```python
from build123d import *

# Parameters (mm, degrees)
SKETCH_1_W          = 47.691438342
SKETCH_1_H          = 48.077140414
EXTRUDE_2_DEPTH     = 10
SKETCH_4_W          = 47.691438342
SKETCH_4_H          = 48.077140414
EXTRUDE_3_DEPTH     = 3
CUT_EXTRUDE_1_DEPTH = 3
SKETCH_6_R          = 11.5
CUT_EXTRUDE_2_DEPTH = 3
CHAMFER_1_SIZE      = 5
SKETCH_7_W          = 26
SKETCH_7_H          = 13
EXTRUDE_4_DEPTH     = 50
SKETCH_8_W          = 20
SKETCH_8_H          = 40
CUT_EXTRUDE_3_DEPTH = 8
SKETCH_9_W          = 20
SKETCH_9_H          = 8
EXTRUDE_5_DEPTH     = 1.93
SKETCH_10_W         = 11.5
SKETCH_10_H         = 13
SKETCH_10_W_2       = 18
EXTRUDE_6_DEPTH     = 25
FILLET_1_R          = 2
SKETCH_11_R         = 2.5
CUT_EXTRUDE_4_DEPTH = 25


with BuildPart() as part:
    # 草图1 → 凸台-拉伸2 (new body)
    with BuildSketch(Plane(origin=(0, 0, 0), x_dir=(1, 0, 0), z_dir=(0, 1, 0))):
        Rectangle(SKETCH_1_W, SKETCH_1_H)
        Polygon((-21.154280829, -15.961429793), (-16.154280829, -20.961429793), (15.845719171, -20.961429793), (20.845719171, -15.961429793), (20.845719171, 16.038570207), (15.845719171, 21.038570207), (-16.154280829, 21.038570207), (-21.154280829, 16.038570207), align=None, mode=Mode.SUBTRACT)
    extrude(amount=EXTRUDE_2_DEPTH)

    # 草图4 → 凸台-拉伸3 (add)
    with BuildSketch(Plane(origin=(0, 10, 0), x_dir=(1, 0, 0), z_dir=(0, 1, 0))):
        Rectangle(SKETCH_4_W, SKETCH_4_H)
    extrude(amount=EXTRUDE_3_DEPTH)

    # 草图5 → 切除-拉伸1 (cut)
    with BuildSketch(Plane.XZ.offset(-10)):
        with BuildLine():
            ThreePointArc((-13.95, -15.5), (-14.403984489, -14.403984489), (-15.5, -13.95))
            Line((-15.5, -13.95), (-15.5, -15.5))
            Line((-15.5, -15.5), (-13.95, -15.5))
        make_face()
        with BuildLine():
            Line((-15.5, -15.5), (-15.5, -13.95))
            ThreePointArc((-15.5, -13.95), (-16.596015511, -16.596015511), (-13.95, -15.5))
            Line((-13.95, -15.5), (-15.5, -15.5))
        make_face()
        with BuildLine():
            ThreePointArc((17.05, -15.5), (16.596015511, -14.403984489), (15.5, -13.95))
            Line((15.5, -13.95), (15.5, -15.5))
            Line((15.5, -15.5), (13.95, -15.5))
            ThreePointArc((13.95, -15.5), (15.5, -17.05), (17.05, -15.5))
        make_face()
        with BuildLine():
            Line((15.5, -15.5), (15.5, -13.95))
            ThreePointArc((15.5, -13.95), (14.403984489, -14.403984489), (13.95, -15.5))
            Line((13.95, -15.5), (15.5, -15.5))
        make_face()
        with BuildLine():
            ThreePointArc((17.05, 15.5), (15.5, 17.05), (13.95, 15.5))
            Line((13.95, 15.5), (15.5, 15.5))
            Line((15.5, 15.5), (15.5, 13.95))
            ThreePointArc((15.5, 13.95), (16.596015511, 14.403984489), (17.05, 15.5))
        make_face()
        with BuildLine():
            Line((15.5, 15.5), (13.95, 15.5))
            ThreePointArc((13.95, 15.5), (14.403984489, 14.403984489), (15.5, 13.95))
            Line((15.5, 13.95), (15.5, 15.5))
        make_face()
        with BuildLine():
            ThreePointArc((-15.5, 13.95), (-14.403984489, 14.403984489), (-13.95, 15.5))
            Line((-13.95, 15.5), (-15.5, 15.5))
            Line((-15.5, 15.5), (-15.5, 13.95))
        make_face()
        with BuildLine():
            Line((-15.5, 15.5), (-13.95, 15.5))
            ThreePointArc((-13.95, 15.5), (-16.596015511, 16.596015511), (-15.5, 13.95))
            Line((-15.5, 13.95), (-15.5, 15.5))
        make_face()
    extrude(amount=-CUT_EXTRUDE_1_DEPTH, mode=Mode.SUBTRACT)

    # 草图6 → 切除-拉伸2 (cut)
    with BuildSketch(Plane(origin=(0, 13, 0), x_dir=(1, 0, 0), z_dir=(0, 1, 0))):
        with Locations(Location((0, 0, 0), (0, 0, 270))):
            Circle(SKETCH_6_R)
    extrude(amount=-CUT_EXTRUDE_2_DEPTH, mode=Mode.SUBTRACT)

    # 倒角1
    chamfer_1_edges = [part.edges().sort_by_distance(p)[0] for p in [
        (23.845719171, 6.5, -24.038570207),
        (23.845719171, 6.5, 24.038570207),
        (-23.845719171, 6.5, 24.038570207),
        (-23.845719171, 6.5, -24.038570207),
    ]]
    chamfer(chamfer_1_edges, length=CHAMFER_1_SIZE)

    # 草图7 → 凸台-拉伸4 (add)
    with BuildSketch(Plane(origin=(0, 0, -24.038570207), x_dir=(-1, 0, 0), z_dir=(0, 0, -1))):
        with Locations((0, 6.5)):
            Rectangle(SKETCH_7_W, SKETCH_7_H)
    extrude(amount=EXTRUDE_4_DEPTH)

    # 草图8 → 切除-拉伸3 (cut)
    with BuildSketch(Plane(origin=(0, 13, 0), x_dir=(1, 0, 0), z_dir=(0, 1, 0))):
        with Locations((0, 54.038570207)):
            Rectangle(SKETCH_8_W, SKETCH_8_H)
    extrude(amount=-CUT_EXTRUDE_3_DEPTH, mode=Mode.SUBTRACT)

    # 草图9 → 凸台-拉伸5 (add)
    with BuildSketch(Plane(origin=(0, 0, -34.038570207), x_dir=(-1, 0, 0), z_dir=(0, 0, -1))):
        with Locations((0, 9)):
            Rectangle(SKETCH_9_W, SKETCH_9_H)
    extrude(amount=EXTRUDE_5_DEPTH)

    # 草图10 → 凸台-拉伸6 (add)
    with BuildSketch(Plane(origin=(13, 0, 0), x_dir=(0, 0, -1), z_dir=(1, 0, 0))):
        with Locations((29.788570207, 6.5)):
            Rectangle(SKETCH_10_W, SKETCH_10_H)
        with Locations((65.038570207, 6.5)):
            Rectangle(SKETCH_10_W_2, SKETCH_10_H)
    extrude(amount=EXTRUDE_6_DEPTH)

    # 圆角1
    fillet_1_edges = [part.edges().sort_by_distance(p)[0] for p in [
        (-13, 0, -49.038570207),
        (13, 6.5, -35.538570207),
        (38, 6.5, -24.038570207),
        (38, 6.5, -35.538570207),
        (13, 6.5, -56.038570207),
        (38, 6.5, -56.038570207),
        (38, 6.5, -74.038570207),
    ]]
    fillet(fillet_1_edges, radius=FILLET_1_R)

    # 草图11 → 切除-拉伸4 (cut)
    with BuildSketch(Plane(origin=(0, 5, 0), x_dir=(1, 0, 0), z_dir=(0, 1, 0))):
        with Locations(Location((0, 64.038570207, 0), (0, 0, 270))):
            Circle(SKETCH_11_R)
        with Locations(Location((0, 49.038570207, 0), (0, 0, 270))):
            Circle(SKETCH_11_R)
    extrude(amount=-CUT_EXTRUDE_4_DEPTH, mode=Mode.SUBTRACT)


solid = part.part
```
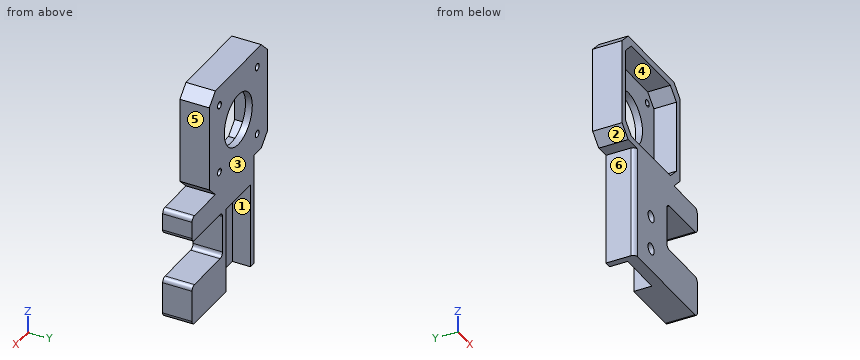
Can you work these out from the model? Positions are in its coordinate system, mm. Face numbers are marked on the shaded views. A direction names the side the tool comes from. Give positions to 0.01 mm unless a question says otherwise; leave off trailing zeros. Loops run counter-clockwise (first coordinate to the right, second up) from the corner with the lowest first, then second, coordinate; pieces in that order, holes last. Notation, with made-up numbers: M 30.25,-18 L 78.25,-18 A26 cw 78.25,21 Z; hole C 12,67.5 d11. An arc over 180 degrees is marked long. Answer in a Markdown table with one row per item.
1. Thinking about a two-plate mould opening in X: for the marked faces 1, 2 and 3, which applies, released by +X, released by -X, zero draft, split by the parting line, or undercut?
Taken from the geometry:
| item | result |
|---|---|
| face 1 | undercut |
| face 2 | released by -X |
| face 3 | zero draft |
2. Which directions (+Z, -Z, +X, -X, +Y, -Y) give clear straight access to the entire face, cutting with the end or side of a thin tool? Please do the marked faces 4, 5 and 6.
Taken from the geometry:
| item | result |
|---|---|
| face 4 | -Y |
| face 5 | +Z, +X, +Y, -Y |
| face 6 | -Z, -X, +Y, -Y |
3. For pin 1 Ø6.5 at (x, y) = (2, 10) entering from -Z; pin 2 Ø1.5 at (y, z) = (9, -55) entering from +X; pin 3 Ø21 at (x, z) = (-4, -0.5) entering from -Y, each with a flat end and sliding along its axis, tell me the tip position at first contact or that it passes through.
Taken from the geometry:
| item | result |
|---|---|
| pin 1 | stops at z = -35.97 |
| pin 2 | stops at x = 13.97 |
| pin 3 | stops at y = 10 |
4. Suppose I cut it at A-A on x = 0. Write out the boundary of the cut face in (y, z).
Taken from the geometry:
| item | result |
|---|---|
| outline | M 0,-74.04 L 5,-74.04 L 5,-66.54 L 0,-66.54 Z; M 0,-61.54 L 5,-61.54 L 5,-51.54 L 0,-51.54 Z; M 0,-46.54 L 5,-46.54 L 5,-35.97 L 13,-35.97 L 13,-11.5 L 10,-11.5 L 10,-21.04 L 0,-21.04 Z; M 0,20.96 L 10,20.96 L 10,11.5 L 13,11.5 L 13,24.04 L 0,24.04 Z |
5. Suppose I cut it at D-D on x = 32.5. Write out the boundary of the cut face in (y, z), plus the area to 4 significant figures.
Taken from the geometry:
| item | result |
|---|---|
| outline | M 0,-74.04 L 13,-74.04 L 13,-56.04 L 0,-56.04 Z; M 0,-35.54 L 13,-35.54 L 13,-24.04 L 0,-24.04 Z |
| area | 383.5 mm² |
6. If I drill on line 1 along X through (y, z) = (10.9, -15.5); line 2 along Z through (x, y) = (-15.5, 11.1); line 3 along X through (y, z) = (2.25, -1.5), over which ranges is the centre line in solid material (lowest first)?
Taken from the geometry:
| item | result |
|---|---|
| line 1 | x = -23.85 to -17.05, -13.95 to 13.95, 17.05 to 23.85 |
| line 2 | z = -24.04 to -17.05, -13.95 to 13.95, 17.05 to 24.04 |
| line 3 | x = -23.85 to -21.15, 20.85 to 23.85 |
7. Suppose I cut it at B-B on z = 0. Write out the boundary of the cut face in (x, y), plus the area to 3 significant figures.
Taken from the geometry:
| item | result |
|---|---|
| outline | M -23.85,0 L -21.15,0 L -21.15,10 L -11.5,10 L -11.5,13 L -23.85,13 Z; M 11.5,10 L 20.85,10 L 20.85,0 L 23.85,0 L 23.85,13 L 11.5,13 Z |
| area | 131 mm² |
